Autodesk Inventor part; units mm, degrees
ref_plane "Work Plane2" through (0, -9.525, 0) normal (0, -1, 0) x (1, 0, 0)
ref_plane "Work Plane1" through (0, 0, -25.4) normal (-1, 0, 0) x (0, 0, 1)
ref_plane "YZ Plane" through (0, 0, 0) normal (1, 0, 0) x (0, 1, 0)
sketch "Sketch1" plane through (0, 0, 0) normal (0, 1, 0) x (-1, 0, 0)
  line L0 (-25.4, 25.4) -> (25.4, 25.4)
  line L1 (25.4, 25.4) -> (25.4, -25.4)
  line L2 (25.4, -25.4) -> (-25.4, -25.4)
  line L3 (-25.4, -25.4) -> (-25.4, 25.4)
  line L4 (-25.4, 25.4) -> (25.4, -25.4) construction
  line L5 (25.4, 25.4) -> (-25.4, -25.4) construction
  point P0 (0, 0)
  dimension "d0" = 50.8
  dimension "d1" = 50.8
extrude "Extrusion1" add sketch "Sketch1" along normal blind 3.1775
sketch "Sketch2" plane through (0, 0, 0) normal (0, -1, 0) x (1, 0, 0)
  circle A0 centre (0, 0) radius 15.875
  dimension "d4" = 31.75
extrude "Extrusion2" cut sketch "Sketch2" against normal blind 3.1775
sketch "Sketch3" plane through (0, 0, 0) normal (0, -1, 0) x (1, 0, 0)
  circle A0 centre (0, 0) radius 19.05
  circle A1 centre (0, 0) radius 15.875
  dimension "d7" = 38.1
extrude "Extrusion3" add sketch "Sketch3" along normal blind 6.35
sketch "Sketch4" plane through (0, -6.35, 0) normal (0, -1, 0) x (1, 0, 0)
  circle A0 centre (0, 0) radius 19.05
  line L0 (-9.35, 12.108) -> (11.15, 12.108) construction
  line L1 (11.15, 12.108) -> (11.15, -14.308) construction
  line L2 (11.15, -14.308) -> (-9.35, -14.308) construction
  line L3 (-9.35, -14.308) -> (-9.35, 12.108) construction
  circle A1 centre (11.15, -14.308) radius 1.016
  circle A2 centre (11.15, 12.108) radius 1.016
  circle A3 centre (-9.35, 12.108) radius 1.016
  circle A4 centre (-9.35, -14.308) radius 1.016
  circle A5 centre (0, 0) radius 15.875
  circle A6 centre (0, 0) radius 19.05
  circle A7 centre (0, 0) radius 15.875
  circle A8 centre (11.15, -14.308) radius 3.175
  circle A9 centre (-9.35, -14.308) radius 3.175
  circle A10 centre (-9.35, 12.108) radius 3.175
  circle A11 centre (11.15, 12.108) radius 3.175
  line L4 (8.3095, 13.5265) -> (8.3095, 17.1422)
  line L5 (-7.0034, 14.2467) -> (-7.0034, 17.716)
  point P0 (11.15, -1.1)
  point P1 (0.9, 12.108)
  point P2 (14.0033, -12.9155)
  point P3 (-12.5247, -14.3539)
  point P4 (-8.1174, -17.234)
  point P5 (9.1025, -16.7346)
  point P6 (-12.0126, 10.3785)
  point P7 (-7.0034, 14.2467)
  point P8 (8.3095, 13.5265)
  point P9 (12.7973, 9.3938)
  point P10 (11.3128, -11.1372)
  point P11 (8.0355, -13.6911)
  point P12 (-6.1902, -14.6184)
  point P13 (-10.9029, -11.5387)
  dimension "d10" = 20.5
  dimension "d11" = 26.416
  dimension "d15" = 2.032
  dimension "d25" = 6.35
  dimension "d26" = 1.1
  dimension "d35" = 0.9
ref_plane "Work Plane2" through (0, -9.525, 0) normal (0, -1, 0) x (1, 0, 0)
sketch "Sketch5" plane through (0, -9.525, 0) normal (0, -1, 0) x (1, 0, 0)
  circle A0 centre (0, 0) radius 15.875
ref_plane "Work Plane1" through (0, 0, -25.4) normal (-1, 0, 0) x (0, 0, 1)
sketch "Sketch6" plane through (0, 0, -25.4) normal (-1, 0, 0) x (0, 0, 1)
  arc A0 (11.2224, 3.1775) -> (10.3522, 0) centre (25.4, -2.413) ccw
  line L0 (9.525, -6.35) -> (9.525, 3.1775)
  line L1 (9.525, 3.1775) -> (41.275, 3.1775)
  line L2 (44.45, 0) -> (6.35, 0)
  line L3 (11.2224, 3.1775) -> (9.525, 3.1775)
  line L4 (9.525, 3.1775) -> (9.525, 0)
  line L5 (9.525, 0) -> (10.3522, 0)
  line L6 (9.525, -9.525) -> (41.275, -9.525)
  line L7 (25.4, -2.413) -> (25.4, -9.525)
  point P0 (25.4, 0)
  point P1 (25.4, -5.969)
  dimension "d21" = 30.48
  dimension "d29" = 7.112
revolve "Revolution1" add sketch "Sketch6" angle 360 about axis through (0, -2.413, 0) along (0, -1, 0)
fillet "Fillet1" radius 1.27 1 edges at (0, 3.1775, 14.1776)
extrude "Extrusion7" add sketch "Sketch4" along normal blind 3.175 contours A0 A11 L4 | L5 A10 A5 A9 A0 | A0 A11 A5 A2 | A5 A2 A11 | A9 A5 A0 | A0 A9 | A10 A5 A3 | A5 A3 A10 | A0 A8 A5 A11 | A9 A5 A8 A0 | A9 A5 | A8 A5 A0 A1 | A0 A1 A8 | A5 A8
sketch "Sketch7" plane through (0, -6.35, 0) normal (0, -1, 0) x (1, 0, 0)
  line L0 (-7.0034, 17.716) -> (-7.0034, 14.2467)
  arc A0 (8.3095, 13.5265) -> (-7.0034, 14.2467) centre (0, 0) ccw
  line L1 (8.3095, 13.5265) -> (8.3095, 17.1422)
  arc A1 (8.3095, 17.1422) -> (-7.0034, 17.716) centre (0, 0) ccw
extrude "Extrusion8" cut sketch "Sketch7" against normal blind 3.175
properties part number "JoystickInsert"
Check sheet for the modelled part. Datum: model origin and axes. Units: mm. A direction names the side the tool comes from. Round coordinates to 2 decimals unless told otherwise and drop trailing zeros. Loops run counter-clockwise (first coordinate to the right, second up) from the corner with the lowest first, then second, coordinate; pieces in that order, holes last. Notation, with made-up numbers: (54, 8) - (96, 8) arc R17 ccw to (96, 12) - close; hole circle Ø5 at (-23.5, 68.25). An arc over 180 degrees is marked (long way). Answer as a JSON object with one key per item and string values. Group by question number.
Q1. Set-up check for faces 1 (the face through (-7.003, -6, 16)), 2 (the face through (0, 2, 25.4)), 3 (the face through (-8, -6.35, 11)), 4 (the face through (9.2, -7.9, -11.8)): record each of +Z, -Z, +X, -X, +Y, -Y from which the full face is reachable in a straight line by a thin tool's end or side.
Q2. Gauge pin test, flat ends, axial feed: P1, Ø4, axis at y = -8, z = 7, coming from the -X side; P2, Ø1.8, axis at x = 11.15, z = 12.108, coming from the -Y side; P3, Ø4, axis at y = -5.5, z = 16, coming from the -X side. Record the tip position at first contact, or that the pin passes through.
Q3. Scan lines: line 1 along Z through (x, y) = (11.15, -8.7); line 2 along Y through (x, z) = (-17, 13.5); line 3 along X through (y, z) = (-9, 12). Record each from-to range of solid material in increasing order. Write a range as [from, to].
Q4. Sectioned sample at A-A, the plane y = -7.75. Count the separate pieces of the cut face and the enclosed holes in it, plus the area to 3 significant figures.
Q5. Mould release check, pull along Y, two halves, no side actions. Record for faces 5 (the face through (12, 3.178, 12)), 6 (the face through (10.401, -7.915, -14.995)), 7 (the face through (-9.8, -6.35, 12.7)), 8 (the face through (12, -6.35, -16)): released by +Y, released by -Y, zero draft, split by the parting line, or undercut.
Q6. Sectioned sample at B-B, the plane z = -20. Enter the section's corners in (x, y).
Solution:
{
 "1": {"face 1": "+Z, -Y", "face 2": "+Z, +X, -X, +Y, -Y", "face 3": "none", "face 4": "-Y"},
 "2": {"P1": "stops at x = -18.38", "P2": "stops at y = -6.35", "P3": "stops at x = -12.92"},
 "3": {"line 1": "z = [-17.48, -15.32], [-13.29, -11.13], [8.93, 11.09], [13.12, 15.45]", "line 2": "y = [0, 3.18]", "line 3": "x = [-14.8, -10.36], [-8.34, -6.18], [7.98, 10.14], [12.16, 14.8]"},
 "4": {"separate pieces": "1", "enclosed holes": "4", "area": "341 mm²"},
 "5": {"face 5": "released by +Y", "face 6": "zero draft", "face 7": "released by -Y", "face 8": "undercut"},
 "6": {"outline": "(-25.4, 0) - (25.4, 0) - (25.4, 3.18) - (-25.4, 3.18) - close"}
}
